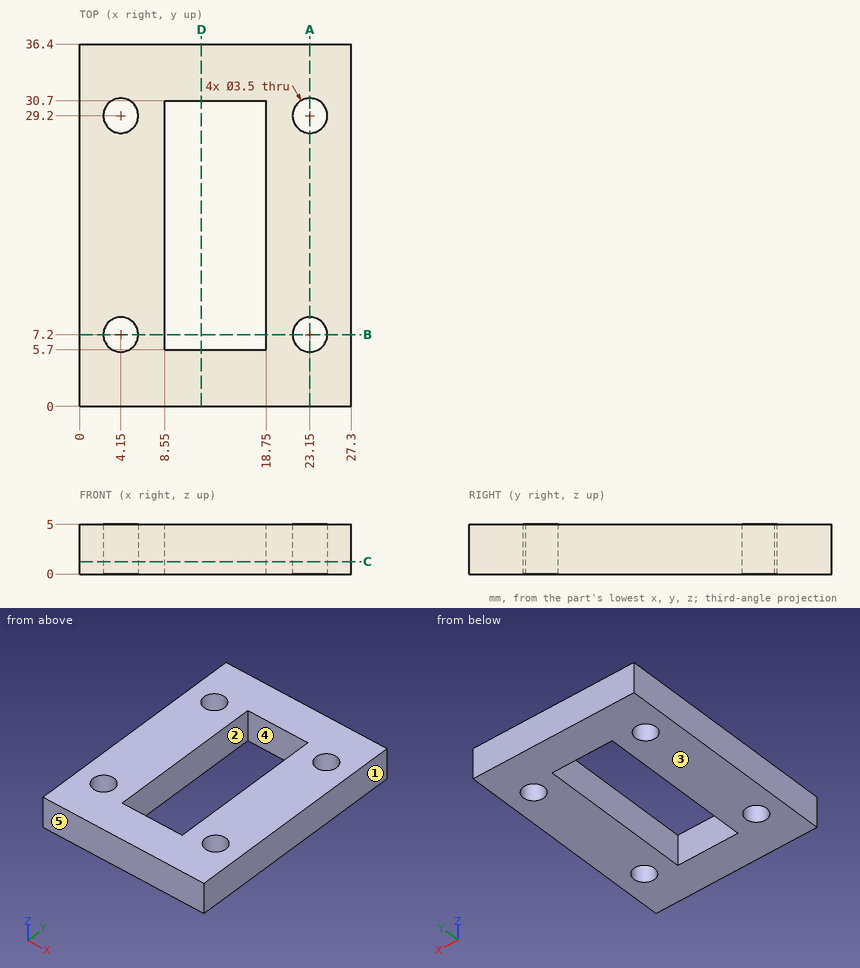
Verification items for this drawing (mm, ordinates from the low corner). A direction names the side the tool comes from. Coordinates: 2 decimals unless noted, no trailing zeros. Order: outer loops, then holes, each group sorted by start corner. A loop starts at its lowest first (then second) coordinate and runs counter-clockwise, first axis right, second up. Notation, with made-up numbers: M 71.25,39 L 100.25,39 A23 ccw 100.25,75 Z; hole C 18.5,66.5 d5. An arc over 180 degrees is marked long. Use CSV: the item, a comma, the result in double quotes.
Item 1: Cross-section at A-A on x = 23.15. Record the cut outline in (y, z).
Returned:
outline,"M 0,0 L 5.45,0 L 5.45,5 L 0,5 Z; M 8.95,0 L 27.45,0 L 27.45,5 L 8.95,5 Z; M 30.95,0 L 36.4,0 L 36.4,5 L 30.95,5 Z"
Item 2: Cross-section at B-B on y = 7.2. Record the cut outline in (x, z), then the cut area to 3 significant figures.
Returned:
outline,"M 0,0 L 2.4,0 L 2.4,5 L 0,5 Z; M 5.9,0 L 8.55,0 L 8.55,5 L 5.9,5 Z; M 18.75,0 L 21.4,0 L 21.4,5 L 18.75,5 Z; M 24.9,0 L 27.3,0 L 27.3,5 L 24.9,5 Z"
area,"50.5 mm2"
Item 3: Cross-section at C-C on z = 1.25. Record the cut outline in (x, y), then the cut area to 3 significant figures.
Returned:
outline,"M 0,0 L 27.3,0 L 27.3,36.4 L 0,36.4 Z; hole C 4.15,7.2 d3.5; hole C 4.15,29.2 d3.5; hole M 8.55,5.7 L 18.75,5.7 L 18.75,30.7 L 8.55,30.7 Z; hole C 23.15,7.2 d3.5; hole C 23.15,29.2 d3.5"
area,"700 mm2"
Item 4: Mould release check, pull along Y, two halves, no side actions. Record for the marked faces 3, 4 and 5: pulls with the +Y half, pulls with the -Y half, needs draft (parallel to the pull), parting line crosses it, or undercut.
Returned:
face 3,"needs draft"
face 4,"undercut"
face 5,"pulls with the -Y half"
Item 5: Thickness scan on line 1 along Y through (x, z) = (4.15, 1.6); line 2 along X through (y, z) = (17, 2.4); line 3 along Y through (x, z) = (12.75, 0.45). Record the ranges inside material, lowest first.
Returned:
line 1,"y = 0 to 5.45, 8.95 to 27.45, 30.95 to 36.4"
line 2,"x = 0 to 8.55, 18.75 to 27.3"
line 3,"y = 0 to 5.7, 30.7 to 36.4"
Item 6: Tool access check on the marked faces 1 and 2. Record the directions out of +Z, -Z, +X, -X, +Y, -Y that give a thin tool (end or side, any length) a straight path to the whole face; none if there is none.
Returned:
face 1,"+Z, -Z, +X, +Y, -Y"
face 2,"+Z, -Z"
Item 7: Cross-section at D-D on x = 12.25. Record the cut outline in (y, z), then the cut area to 3 significant figures.
Returned:
outline,"M 0,0 L 5.7,0 L 5.7,5 L 0,5 Z; M 30.7,0 L 36.4,0 L 36.4,5 L 30.7,5 Z"
area,"57.0 mm2"
